```python
from build123d import *

# Parameters (mm, degrees)
F0_W     = 68.6
F0_H     = 53.2
F0_R     = 1.4
F0_H_2   = 3
F1_DEPTH = 2
F2_DEPTH = 12
F0_H_3   = 1
F3_DEPTH = 6
F4_DEPTH = 8


with BuildPart() as f1:
    # F0 (on Top) → F1 (new body)
    with BuildSketch(Plane.XY):
        with Locations((134.3, 46.6)):
            Rectangle(F0_W, F0_H)
        with Locations((114, 22.5)):
            Circle(F0_R, mode=Mode.SUBTRACT)
        with Locations((166.1, 27.6)):
            Circle(F0_R, mode=Mode.SUBTRACT)
        with Locations((166.1, 55.5)):
            Circle(F0_R, mode=Mode.SUBTRACT)
        with Locations((115.3, 70.7)):
            Circle(F0_R, mode=Mode.SUBTRACT)
        with Locations((134.3, 74.7)):
            Rectangle(F0_W, F0_H_2)
        Polygon((168.6, 20), (100, 20), (50.6, 20), (50.6, 18), (168.6, 18), align=None)
        Polygon((100, 20), (100, 73.2), (100, 76.2), (100, 77.2), (50.6, 77.2), (50.6, 20), align=None)
    extrude(amount=F1_DEPTH)

    # F0 (on Top) → F2 (join)
    with BuildSketch(Plane.XY):
        with Locations((115.3, 70.7)):
            Circle(F0_R)
        with Locations((166.1, 55.5)):
            Circle(F0_R)
        with Locations((166.1, 27.6)):
            Circle(F0_R)
        with Locations((114, 22.5)):
            Circle(F0_R)
    extrude(amount=F2_DEPTH)

    # F0 (on Top) → F3 (join)
    with BuildSketch(Plane.XY):
        with Locations((134.3, 76.7)):
            Rectangle(F0_W, F0_H_3)
    extrude(amount=F3_DEPTH)

    # F0 (on Top) → F4 (join)
    with BuildSketch(Plane.XY):
        Polygon((168.6, 12), (168.6, 18), (50.6, 18), (50.6, 12), (60.6, 12), (58.85, 15.5), (62.35, 15.5), (65.85, 15.5), (64.1, 12), (155.1, 12), (153.35, 15.5), (156.85, 15.5), (160.35, 15.5), (158.6, 12), align=None)
    extrude(amount=F4_DEPTH)


solid = f1.part
```
Model file for the job. Use its own axes, mm. A direction names the side the tool comes from. Coordinates: 2 decimals unless noted, no trailing zeros. Loops run counter-clockwise (first coordinate to the right, second up) from the corner with the lowest first, then second, coordinate; pieces in that order, holes last. Notation, with made-up numbers: (71.25, -20.75) - (130.25, -20.75) arc R14 ccw to (130.25, -6.75) - close; hole circle Ø4 at (22, -27). An arc over 180 degrees is marked (long way). Write item = value, one per line. Start each with the question number.
Item 1: Drop flat-ended pins along their axis: pin 1 Ø1.8 at (x, z) = (83.5, 4.5) entering from +Y; pin 2 Ø6.5 at (x, y) = (132, 15) entering from +Z; pin 3 Ø0.5 at (x, y) = (120.5, 76.5) entering from +Z. Give the stop position or say it passes through.
Item 2: Saw through at D-D, the plane z = 10. List the corners of the cut face in (x, y), then the cut area to 3 significant figures.
Item 3: Saw through at A-A, the plane z = 4. List the corners of the cut face in (x, y).
Item 4: Saw through at C-C, the plane y = 22.5. List the corners of the cut face in (x, z), then the cut area to 3 significant figures.
Item 5: 3-axis set-ups, long thin cutter, end or side, ignore diameter. For faces 1 (the face through (166, 28, 12)), 2 (the face through (112.89, 21.65, 6.93)): which of +Z, -Z, +X, -X, +Y, -Y reach the whole face in a straight line?
Item 6: Saw through at B-B, the plane x = 118. List the corners of the cut face in (y, z).
Item 7: Pull direction Y, two halves, no side cores. Call faces 3 (the face through (109, 12, 4)), 4 (the face through (109, 45, 0)), 5 (the face through (134, 76.2, 4)), 6 (the face through (154.237, 13.726, 3.944)): +Y half, -Y half, draft (parallel to the pull), parting line (faces both ways), or undercut.
Item 8: Wall check: probe 1 along Y at (x, z) = (148, 5.75); probe 2 along Z at (x, y) = (134.5, 16.5); probe 3 along Z at (x, y) = (96, 58.5). Give the ranges that are in metal, low to high. Write a range as [from, to].
Answers:
q1.pin_1 = 18
q1.pin_2 = 8
q1.pin_3 = 6
q2.outline = circle Ø2.8 at (114, 22.5); circle Ø2.8 at (115.3, 70.7); circle Ø2.8 at (166.1, 27.6); circle Ø2.8 at (166.1, 55.5)
q2.area = 24.6 mm2
q3.outline = (50.6, 12) - (60.6, 12) - (58.85, 15.5) - (65.85, 15.5) - (64.1, 12) - (155.1, 12) - (153.35, 15.5) - (160.35, 15.5) - (158.6, 12) - (168.6, 12) - (168.6, 18) - (50.6, 18) - close; (100, 76.2) - (168.6, 76.2) - (168.6, 77.2) - (100, 77.2) - close; circle Ø2.8 at (114, 22.5); circle Ø2.8 at (115.3, 70.7); circle Ø2.8 at (166.1, 27.6); circle Ø2.8 at (166.1, 55.5)
q4.outline = (50.6, 0) - (168.6, 0) - (168.6, 2) - (115.4, 2) - (115.4, 12) - (112.6, 12) - (112.6, 2) - (50.6, 2) - close
q4.area = 264 mm2
q5.face_1 = +Z, +X, -X, +Y, -Y
q5.face_2 = +Z
q6.outline = (12, 0) - (77.2, 0) - (77.2, 6) - (76.2, 6) - (76.2, 2) - (18, 2) - (18, 8) - (12, 8) - close
q7.face_3 = -Y half
q7.face_4 = draft
q7.face_5 = undercut
q7.face_6 = undercut
q8.probe_1 = [12, 18], [76.2, 77.2]
q8.probe_2 = [0, 8]
q8.probe_3 = [0, 2]
